Verification items for the finished model (mm, model axes). A direction names the side the tool comes from. Coordinates: 2 decimals unless noted, no trailing zeros. Order: outer loops, then holes, each group sorted by start corner. A loop starts at its lowest first (then second) coordinate and runs counter-clockwise, first axis right, second up. Notation, with made-up numbers: M 0,-32.75 L 56,-32.75 A3 ccw 56,-28.75 Z; hole C 53.5,-18 d3. An arc over 180 degrees is marked long. Write item = value, one per line.
Autodesk Inventor part; units mm, degrees
ref_plane "Work Plane1" through (1.525, 0, 0) normal (0, 0, 1) x (1, 0, 0)
ref_plane "YZ Plane" through (0, 0, 0) normal (1, 0, 0) x (0, 1, 0)
ref_plane "XZ Plane" through (0, 0, 0) normal (0, 1, 0) x (-1, 0, 0)
sketch "Sketch1" plane through (0, 0, 0) normal (0, 0, 1) x (1, 0, 0)
  line L0 (0, 14.095) -> (0, 10)
  line L1 (54, 10) -> (100, 10)
  line L2 (100, 10) -> (100, 0)
  line L3 (100, 0) -> (-0.8001, 0)
  line L4 (-20.9601, 0) -> (120.16, 0)
  line L5 (-0.8001, 0) -> (-0.8001, 14.095)
  line L6 (-0.8001, 14.095) -> (0, 14.095)
  line L7 (54, 10) -> (52.773, 10)
  line L8 (52.773, 10) -> (0, 10)
  line L9 (0, -2.819) -> (0, 16.914)
  dimension "d0" = 100
  dimension "d1" = 46
  dimension "d2" = 20
  dimension "d9" = 0.8001
  dimension "d10" = 28.19
  dimension "d13" = 1.227
  dimension "d14" = 20
revolve "Body" add sketch "Sketch1" angle 360 about axis through (100, 0, 0) along (-1, 0, 0)
sketch "Sketch2" plane through (-0.8001, 0, 0) normal (-1, 0, 0) x (0, 0, 1)
  line L0 (0, 17.3205) -> (15, 8.6603)
  line L1 (15, 8.6603) -> (15, -8.6603)
  line L2 (15, -8.6603) -> (0, -17.3205)
  line L3 (0, -17.3205) -> (-15, -8.6603)
  line L4 (-15, -8.6603) -> (-15, 8.6603)
  line L5 (-15, 8.6603) -> (0, 17.3205)
  point P0 (0, 0)
  point P1 (0, 0)
  dimension "d11" = 30
extrude "Head" add sketch "Sketch2" along normal blind 11.7
sketch "Sketch4" plane through (0, 0, 0) normal (0, 0, 1) x (1, 0, 0)
  line L0 (-12.5001, 15) -> (-12.5001, 17.3205)
  line L1 (-12.5001, 17.3205) -> (-11.1604, 17.3205)
  line L2 (-11.1604, 17.3205) -> (-12.5001, 15)
  line L3 (-14.8401, 0) -> (1.5399, 0)
  line L4 (-0.8001, 17.3205) -> (-12.5001, 17.3205)
  line L5 (-12.5001, 8.6603) -> (-12.5001, 17.3205)
  dimension "d5" = 30
  dimension "d19" = 30
revolve "Chamfer1" cut sketch "Sketch4" angle 360 about axis through (-10, 0, 0) along (1, 0, 0)
thread "Thread"
chamfer "Chamfer2" distance 1.2269 distance2 1.227 1 edges at (100, -10, 0) measured on face at (100, 2.4562, 0.99)
ref_plane "Work Plane1" through (1.525, 0, 0) normal (0, 0, 1) x (1, 0, 0)
equation "\"d0\" = NLG"
equation "\"d1\" = GEL"
equation "\"d2\" = GD"
equation "\"d10\" = SD2"
equation "\"d14\" = BDM"
equation "\"d11\" = SW"
equation "\"d3\" = KOH - SD"
equation "\"d5\" = ANG1"
equation "\"d19\" = SW0"
equation "\"d15\" = GEL"
equation "\"d6\" = -0.5 * SPD + 0.5 * GD"
equation "\"NLG\" = 100"
equation "\"GD\" = NND"
equation "\"BDM\" = NND"
equation "\"KOH\" = 12.5"
equation "\"GEL\" = 46"
equation "\"SW\" = 30"
equation "\"SW0\" = SW"
equation "\"SPD\" = NND - 1.2269 * PTC"
equation "\"SD2\" = 28.19"
equation "\"SD\" = 0.8"
equation "\"ANG1\" = 30deg"
equation "\"GAL\" = 0.61345 * PTC"
equation "\"GUL\" = 0.61345 * PTC"
equation "\"RR\" = 0.8"
equation "\"GD1\" = THREADDIA - 1.2269 * PTC"
equation "\"SDH\" = SD2"
equation "\"TOA\" = 30deg"
equation "\"PTC\" = 2"
equation "\"E0\" = 1.155 * SW"
properties part number "ISO 8765 - M20 x 2 x 100" material "Stainless Steel, 440C"
Item 1: Sectioned sample at A-A, the plane x = 15. Enter the section's corners in (y, z).
Report:
outline = C 0,0 d20
Item 2: Release check for a two-part mould opening along Y. For faces 3 (the cylindrical face through (50.08, -2.17, -9.76)), 4 (the flat face through (0, -10, 3)), 5 (the conical face through (-12.174, -7.749, 13.498)) record: pulls with the +Y half, pulls with the -Y half, needs draft (parallel to the pull), parting line crosses it, or undercut.
Report:
face_3 = parting line crosses it
face_4 = needs draft
face_5 = pulls with the -Y half
Item 3: Gauge pin test, flat ends, axial feed: pin 1 (8 mm diameter, centred on x = 14, y = 7.5, fed in from +Z); pin 2 (10 mm diameter, centred on x = 25.5, z = -2.5, fed in from +Y); pin 3 (1.5 mm diameter, centred on x = 55.5, z = -5, fed in from -Y). Record the tip position at first contact, or that the pin passes through.
Report:
pin_1 = 9.37
pin_2 = 10
pin_3 = -9.05
Item 4: Scan lines: L1, parallel to X at y = -13, z = 4; L2, parallel to Y at x = 69.5, z = -0.5; L3, parallel to Z at x = 87.5, y = -4.5. Record each from-to range of solid material in increasing order. Write a range as from..to.
Report:
L1 = -12.5..0
L2 = -9.99..9.99
L3 = -8.93..8.93
Item 5: Tool access check on faces 1 (the flat face through (-0.8, -14, -3)), 2 (the conical face through (-12.174, 15.564, -0.038)). Record the directions out of +Z, -Z, +X, -X, +Y, -Y that give a thin tool (end or side, any length) a straight path to the whole face; none if there is none.
Report:
face_1 = +X
face_2 = -X, +Y
